Geometry check sheet. Reference: the model listing, model coordinates, mm. Face numbers are marked on the shaded views. A direction names the side the tool comes from. Coordinates: 2 decimals unless noted, no trailing zeros. Write each loop counter-clockwise with the first axis right and the second up, starting at its lowest first coordinate (ties: lowest second). Pieces come first, ordered by that corner, then holes. Notation, with made-up numbers: (85, 18) -> (113, 18) arc R38 ccw to (113, 56) -> close; hole circle Ø3 at (-34, -40). An arc over 180 degrees is marked (long way). Answer in a Markdown table with one row per item. Add a question column.
1. Cross-section at B-B on y = 41. Give the number of separate pieces and of enclosed holes in the cut face, and give its area (3 significant figures).
2. Set-up check for the marked faces 5 and 6: record each of +Z, -Z, +X, -X, +Y, -Y from which the full face is reachable in a straight line by a thin tool's end or side.
3. Depth check by flat-ended pin: P1, Ø1, axis at y = 31, z = -7, coming from the -X side; P2, Ø3, axis at x = -17, z = -14, coming from the +Y side; P3, Ø3, axis at x = 9, y = 41.5, coming from the -Z side; P4, Ø3, axis at x = 3.62, y = 54.61, coming from the -Z side. Enter the tip coordinate at first touch or a pass-through.
4. Mould release check, pull along X, two halves, no side actions. Record for the marked faces 1, 2, 3 and 4: pulls with the +X half, pulls with the -X half, needs draft (parallel to the pull), parting line crosses it, or undercut.
5. Scan lines: L1, parallel to X at y = 43, z = -2.5; L2, parallel to X at y = 26.5, z = 1; L3, parallel to Z at x = -5, y = 37. Record each from-to range of solid material in increasing order. Write a range as from..to.
6. Cross-section at A-A on y = 13. Record the cut outline in (x, z), and give its area (3 significant figures).
```python
from build123d import *

# Parameters (mm, degrees)
SKETCH1_R                  = 26.8
MAIN_BODY_EXTRUDE_DEPTH    = 41.945
ANGLED_EXTRUDE_OUTLINE_R   = 26.8
ANGLED_EXTRUDE_DEPTH       = 6.012203303
ANGLED_START               = 44.670962752
ANGLED_EXTRUDE_2_OUTLINE_W = 56
ANGLED_EXTRUDE_2_OUTLINE_H = 56
ANGLED_EXTRUDE_2_DEPTH     = 7.329037248
SKETCH8_R                  = 16.325
ATTACHMENT_EXTRUDE_DEPTH   = 22.5
SKETCH11_R                 = 12.7625
SKETCH11_R_2               = 11.2625
TUBING_HOLE_DEPTH          = 45
SKETCH13_R                 = 2
BOLT_HOLE_DEPTH            = 25
SKETCH14_W                 = 34.35
SKETCH14_H                 = 34.35
CUT_EXTRUDE3_DEPTH         = 4
CUT_EXTRUDE4_DEPTH         = 2
SKETCH16_W                 = 23.74
SKETCH16_H                 = 28.35
CUT_EXTRUDE5_DEPTH         = 3.5
CUT_EXTRUDE12_REACH        = 74.294
SKETCH36_W                 = 2
SKETCH36_H                 = 3
FILLET3_R                  = 5
SKETCH32_R                 = 17.343535691
CUT_EXTRUDE10_DEPTH        = 5


with BuildPart() as part:
    # Sketch1 → Main Body Extrude (new body)
    with BuildSketch(Plane(origin=(0, 0, 0), x_dir=(1, 0, 0), z_dir=(0, 1, 0))):
        with Locations(Location((0, 0, 0), (0, 0, 270))):
            Circle(SKETCH1_R)
    extrude(amount=MAIN_BODY_EXTRUDE_DEPTH)

    # Angled Extrude: read off the stored shape, not the designer's step
    # Angled Extrude outline → Angled Extrude (add)
    with BuildSketch(Plane(origin=(0, 41.945, 0), x_dir=(1, 0, 0), z_dir=(0, 1, 0))):
        Circle(ANGLED_EXTRUDE_OUTLINE_R)
    extrude(amount=ANGLED_EXTRUDE_DEPTH)

    # Angled Extrude 2 outline → Angled Extrude 2 (cut)
    with BuildSketch(Plane(origin=(0, 0, 0), x_dir=(0.9937679191605965, -0.11146893220632507, 0), z_dir=(0.11146893220632506, 0.9937679191605965, 0)).offset(ANGLED_START)):
        with Locations((-5, 0)):
            Rectangle(ANGLED_EXTRUDE_2_OUTLINE_W, ANGLED_EXTRUDE_2_OUTLINE_H)
    extrude(amount=ANGLED_EXTRUDE_2_DEPTH, mode=Mode.SUBTRACT)

    # Sketch8 → Attachment Extrude (add)
    with BuildSketch(Plane(origin=(4.979424519, 44.392569701, 0), x_dir=(0.9937679191605964, -0.11146893220632542, 0), z_dir=(0.11146893220632542, 0.9937679191605964, 0))):
        with Locations(Location((-2.486871931, 0, 0), (0, 0, 180))):
            Circle(SKETCH8_R)
    extrude(amount=ATTACHMENT_EXTRUDE_DEPTH)

    # Sketch11 → Tubing Hole (cut)
    with BuildSketch(Plane(origin=(7.487475493, 66.752347882, 0), x_dir=(0.9937679191605964, -0.11146893220632542, 0), z_dir=(0.11146893220632542, 0.9937679191605964, 0))):
        with Locations(Location((-2.486871931, 0, 0), (0, 0, 180))):
            Circle(SKETCH11_R)
        with Locations(Location((-2.486871931, 0, 0), (0, 0, 180))):
            Circle(SKETCH11_R_2, mode=Mode.SUBTRACT)
    extrude(amount=-TUBING_HOLE_DEPTH, mode=Mode.SUBTRACT)

    # Sketch13 → Bolt Hole (cut, symmetric)
    with BuildSketch(Plane.XY):
        with Locations((3.622740297, 54.607457852)):
            Circle(SKETCH13_R)
    extrude(amount=BOLT_HOLE_DEPTH, both=True, mode=Mode.SUBTRACT)

    # Sketch14 → Cut-Extrude3 (cut)
    with BuildSketch(Plane.XZ):
        Rectangle(SKETCH14_W, SKETCH14_H)
    extrude(amount=-CUT_EXTRUDE3_DEPTH, mode=Mode.SUBTRACT)

    # Sketch15 → Cut-Extrude4 (cut)
    with BuildSketch(Plane.XZ.offset(-4)):
        with BuildLine():
            ThreePointArc((-6.675, -12.175), (-5.175, -13.675), (-3.675, -12.175))
            Line((-3.675, -12.175), (-6.675, -12.175))
        make_face()
        with BuildLine():
            Line((-6.675, -12.175), (-3.675, -12.175))
            ThreePointArc((-3.675, -12.175), (-5.175, -10.675), (-6.675, -12.175))
        make_face()
        with BuildLine():
            ThreePointArc((-10.675, 0), (-11.114339828, 1.060660172), (-12.175, 1.5))
            Line((-12.175, 1.5), (-12.175, -1.5))
            ThreePointArc((-12.175, -1.5), (-11.114339828, -1.060660172), (-10.675, 0))
        make_face()
        with BuildLine():
            Line((-12.175, -1.5), (-12.175, 1.5))
            ThreePointArc((-12.175, 1.5), (-13.675, 0), (-12.175, -1.5))
        make_face()
        with BuildLine():
            ThreePointArc((-6.675, 12.175), (-5.175, 10.675), (-3.675, 12.175))
            Line((-3.675, 12.175), (-6.675, 12.175))
        make_face()
        with BuildLine():
            Line((-6.675, 12.175), (-3.675, 12.175))
            ThreePointArc((-3.675, 12.175), (-5.175, 13.675), (-6.675, 12.175))
        make_face()
    extrude(amount=-CUT_EXTRUDE4_DEPTH, mode=Mode.SUBTRACT)

    # Sketch16 → Cut-Extrude5 (cut)
    with BuildSketch(Plane.XZ.offset(-4)):
        with Locations((-2.305, 0)):
            Rectangle(SKETCH16_W, SKETCH16_H)
    extrude(amount=-CUT_EXTRUDE5_DEPTH, mode=Mode.SUBTRACT)

    # Fillet1: read off the stored shape, not the designer's step
    # Fillet1 outline → Fillet1 (revolve, cut)
    with BuildSketch(Plane.XY):
        with BuildLine():
            ThreePointArc((26.8, 2), (26.214213562, 0.585786438), (24.8, 0))
            Line((24.8, 0), (26.8, 0))
            Line((26.8, 0), (26.8, 2))
        make_face()
    revolve(axis=Axis((0, 0, 0), (0, 1, 0)), mode=Mode.SUBTRACT)

    # Cut-Extrude12: up to this plane
    cut_extrude12_end = Plane(origin=(5.016101949, 67.029556841, 0), z_dir=(0.11146893220632542, 0.9937679191605964, 0))
    # Sketch36 → Cut-Extrude12 (cut, up to the surface)
    with BuildSketch(Plane.XZ.offset(-7.5), mode=Mode.PRIVATE) as cut_extrude12_sk1:
        with Locations((7.065, 3)):
            Rectangle(SKETCH36_W, SKETCH36_H)
    cut_extrude12_tool1 = split(extrude(cut_extrude12_sk1.sketch, amount=CUT_EXTRUDE12_REACH, dir=(0.069756473744, 0.99756405026, 0), mode=Mode.PRIVATE), bisect_by=cut_extrude12_end, keep=Keep.BOTH, mode=Mode.PRIVATE)
    add(cut_extrude12_tool1.solids().sort_by_distance((7.065, 7.5, 3))[0], mode=Mode.SUBTRACT)
    # Sketch36 → Cut-Extrude12 (cut, up to the surface)
    with BuildSketch(Plane.XZ.offset(-7.5), mode=Mode.PRIVATE) as cut_extrude12_sk2:
        with Locations((7.065, -3)):
            Rectangle(SKETCH36_W, SKETCH36_H)
    cut_extrude12_tool2 = split(extrude(cut_extrude12_sk2.sketch, amount=CUT_EXTRUDE12_REACH, dir=(0.069756473744, 0.99756405026, 0), mode=Mode.PRIVATE), bisect_by=cut_extrude12_end, keep=Keep.BOTH, mode=Mode.PRIVATE)
    add(cut_extrude12_tool2.solids().sort_by_distance((7.065, 7.5, -3))[0], mode=Mode.SUBTRACT)

    # Fillet3
    fillet3_edges = [part.edges().sort_by_distance(p)[0] for p in [
        (18.731312255, 42.850048342, 0),
    ]]
    fillet(fillet3_edges, radius=FILLET3_R)

    # Sketch32 → Cut-Extrude10 (cut)
    with BuildSketch(Plane(origin=(7.487475493, 66.752347882, 0), x_dir=(0.9937679191605965, -0.11146893220632544, 0), z_dir=(0.11146893220632544, 0.9937679191605965, 0))):
        with Locations((-2.464764356, 0)):
            Circle(SKETCH32_R)
    extrude(amount=-CUT_EXTRUDE10_DEPTH, mode=Mode.SUBTRACT)


solid = part.part
```
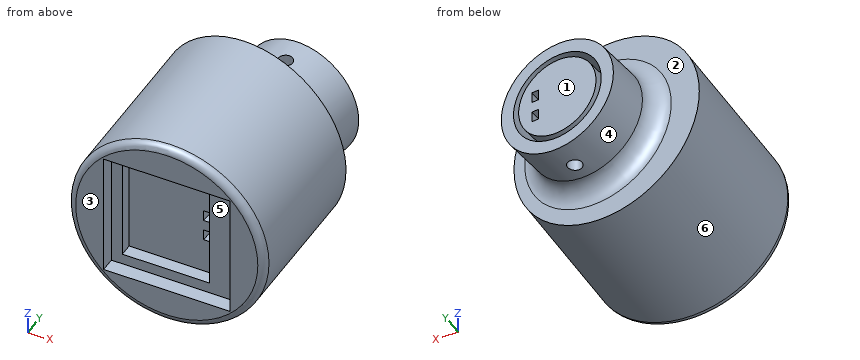
Results found:
| question | item | result |
|---|---|---|
| 1 | separate pieces | 2 |
| 1 | enclosed holes | 3 |
| 1 | area | 2,130 mm^2 |
| 2 | face 5 | -Y |
| 2 | face 6 | +Y, -Y |
| 3 | P1 | stops at x = -26 |
| 3 | P2 | stops at y = 47.03 |
| 3 | P3 | stops at z = -25.73 |
| 3 | P4 | passes through |
| 4 | face 1 | pulls with the +X half |
| 4 | face 2 | undercut |
| 4 | face 3 | needs draft |
| 4 | face 4 | parting line crosses it |
| 5 | L1 | x = -26.68..-10.27, -8.73..8.55, 10.55..13.37, 14.91..21.51 |
| 5 | L2 | x = -26.78..-12.33, -10.82..11.76, 13.27..26.78 |
| 5 | L3 | z = -26.33..-10.92, -9.12..9.12, 10.92..26.33 |
| 6 | outline | circle Ø53.6 at (0, 0); hole (6.45, -4.5) -> (8.45, -4.5) -> (8.45, -1.5) -> (6.45, -1.5) -> close; hole (6.45, 1.5) -> (8.45, 1.5) -> (8.45, 4.5) -> (6.45, 4.5) -> close |
| 6 | area | 2,240 mm^2 |
